```python
from build123d import *

# Parameters (mm, degrees)
FILLET_1_R          = 0.2
CHAMFER_1_SIZE      = 0.2
SKETCH_3_W          = 0.5
SKETCH_3_H          = 0.25
CUT_EXTRUDE_1_DEPTH = 2


with BuildPart() as part:
    # 草图1 → 旋转1 (revolve)
    with BuildSketch(Plane.XY):
        Polygon((-8.5, 0), (-8.5, 3), (-5.5, 3), (-5.5, 1.5), (4.5, 1.5), (4.5, 1.25), (8.5, 1.25), (8.5, 0), align=None)
    revolve(axis=Axis((-8.5, 0, 0), (1, 0, 0)))

    # 圆角1
    fillet_1_edges = [part.edges().sort_by_distance(p)[0] for p in [
        (-5.5, -3, 0),
        (-8.5, -3, 0),
    ]]
    fillet(fillet_1_edges, radius=FILLET_1_R)

    # 倒角1
    chamfer_1_edges = [part.edges().sort_by_distance(p)[0] for p in [
        (8.5, -1.25, 0),
    ]]
    chamfer(chamfer_1_edges, length=CHAMFER_1_SIZE)

    # 草图3 → 切除-旋转1 (revolve, cut)
    with BuildSketch(Plane.XY):
        with Locations((4.75, 1.125)):
            Rectangle(SKETCH_3_W, SKETCH_3_H)
    revolve(axis=Axis((4.5, 0, 0), (1, 0, 0)), mode=Mode.SUBTRACT)

    # 草图4 → 切除-拉伸1 (cut)
    with BuildSketch(Plane.ZY.offset(8.5)):
        Polygon((1.732050808, 0), (0.866025404, 1.5), (-0.866025404, 1.5), (-1.732050808, 0), (-0.866025404, -1.5), (0.866025404, -1.5), align=None)
    extrude(amount=-CUT_EXTRUDE_1_DEPTH, mode=Mode.SUBTRACT)


solid = part.part
```
The listing builds one solid part. Answer for the finished solid, in the listing's coordinates (mm). A direction names the side the tool comes from. Coordinates: 2 decimals unless noted, no trailing zeros. Write each loop counter-clockwise with the first axis right and the second up, starting at its lowest first coordinate (ties: lowest second). Pieces come first, ordered by that corner, then holes. Notation, with made-up numbers: M -18,63 L 38,63 A13 ccw 38,87 Z; hole C -38,-14.75 d3. An arc over 180 degrees is marked long. Use a Markdown table: item, result. Add a question column.
1. For a pull along X with two mould halves and no side action, classify faces 1 (the flat face through (-7.514, 0.76, -1.293)), 2 (the flat face through (8.5, 0, 0)), 3 (the cylindrical face through (4.754, -0.217, -0.976)) as +X half, -X half, draft (parallel to the pull), parting line (faces both ways), or undercut.
2. Given P1, Ø1.5, axis at y = -0.5, z = 0, coming from the -X side, flat-ended and moving along its own axis, determine where the tip first touches the part or whether it passes through.
3. Section B-B (x = 6.25) is taken. Give the vertices of the cut face in (y, z), plus the area to 3 significant figures.
4. Section A-A (z = 0) is taken. Give the vertices of the cut face in (x, y).
5. Section C-C (x = 0.5) is taken. Give the vertices of the cut face in (y, z).
6. Straight lines are drawn through the part: line 1 along X through (y, z) = (0.25, -2); line 2 along Z through (x, y) = (2.5, 0); line 3 along Z through (x, y) = (6, 0.75). For each, find the intervals that lie inside material, in ascending order. Write a range as [from, to].
7. Which of the six approach directions +Z, -Z, +X, -X, +Y, -Y give full straight-line access (tool end or side, diameter ignored) to faces 4 (the flat face through (-8.5, -1.21, -1.21)), 5 (the flat face through (-7.514, -0.74, -1.305)), 6 (the cylindrical face through (-0.43, -1.5, 0.07))?
Data:
| question | item | result |
|---|---|---|
| 1 | face 1 | draft |
| 1 | face 2 | +X half |
| 1 | face 3 | undercut |
| 2 | P1 | stops at x = -6.5 |
| 3 | outline | C 0,0 d2.5 |
| 3 | area | 4.91 mm2 |
| 4 | outline | M -8.5,-2.8 A0.2 ccw -8.3,-3 L -5.7,-3 A0.2 ccw -5.5,-2.8 L -5.5,-1.5 L 4.5,-1.5 L 4.5,-1 L 5,-1 L 5,-1.25 L 8.3,-1.25 L 8.5,-1.05 L 8.5,1.05 L 8.3,1.25 L 5,1.25 L 5,1 L 4.5,1 L 4.5,1.5 L -5.5,1.5 L -5.5,2.8 A0.2 ccw -5.7,3 L -8.3,3 A0.2 ccw -8.5,2.8 L -8.5,1.5 L -6.5,1.5 L -6.5,-1.5 L -8.5,-1.5 Z |
| 5 | outline | C 0,0 d3 |
| 6 | line 1 | x = [-8.5, -5.5] |
| 6 | line 2 | z = [-1.5, 1.5] |
| 6 | line 3 | z = [-1, 1] |
| 7 | face 4 | +Z, -Z, -X, +Y, -Y |
| 7 | face 5 | -X |
| 7 | face 6 | +X |
